Work out the finished part from the listing and answer in its coordinate system (mm). Face numbers are marked on the shaded views. A direction names the side the tool comes from. Give positions to 0.01 mm unless a question says otherwise; leave off trailing zeros. Write each loop counter-clockwise with the first axis right and the second up, starting at its lowest first coordinate (ties: lowest second). Pieces come first, ordered by that corner, then holes.
1) Given pin 1 Ø3 at (x, z) = (-38.5, -9) entering from -Y; pin 2 Ø3 at (x, z) = (14, 1) entering from +Y; pin 3 Ø0.5 at (y, z) = (13.5, -7.5) entering from -X; pin 4 Ø3 at (x, z) = (-38, 8) entering from -Y, each flat-ended and moving along its own axis, determine where each tip first touches the part or whether it passes through.
2) Determine the mould class of the marked faces 1, 2 and 3 for opening direction Z: pulls with the +Z half, pulls with the -Z half, needs draft (parallel to the pull), parting line crosses it, or undercut.
3) Find section B-B (z = 11). Determine the outline of the cut face in (x, y).
4) Find section A-A (y = 2.5). Determine the outline of the cut face in (x, z), plus the area to 3 significant figures.
5) A tool of negligible diameter and unlimited length cuts with its end or side. For the marked faces 4 and 5, from which of +Z, -Z, +X, -X, +Y, -Y can it reach the whole face along a straight path? Write none if from no direction.
6) Find section D-D (z = -8). Determine the outline of the cut face in (x, y), plus the area to 3 significant figures.
7) Straight lines are drawn through the part: probe 1 along X at (y, z) = (2.1, 8); probe 2 along Z at (x, y) = (24, 4); probe 3 along Y at (x, z) = (-5, 2). For each, find the intervals that lie inside material, in ascending order.
8) Find section C-C (x = 10). Determine the outline of the cut face in (y, z).
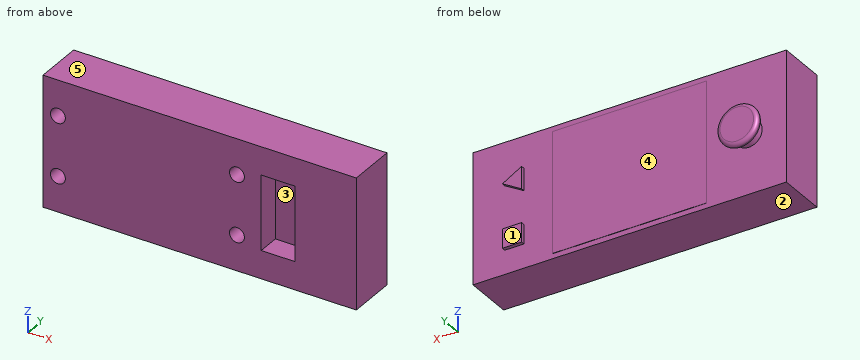
```python
from build123d import *

# Parameters (mm, degrees)
SKETCH_1_W          = 84
SKETCH_1_H          = 35
EXTRUDE_1_DEPTH     = 13
SKETCH_2_R          = 3.636879205
EXTRUDE_2_DEPTH     = 3
EXTRUDE_2_TAPER     = 10
SKETCH_2_3_W        = 5.141866658
SKETCH_2_3_H        = 5.141866659
EXTRUDE_3_DEPTH     = 1
SKETCH_2_4_W        = 41.257358664
SKETCH_2_4_H        = 32.32030471
EXTRUDE_4_DEPTH     = 0.1
SKETCH_4_R          = 5.5
EXTRUDE_5_DEPTH     = 2
FILLET_1_R          = 1
SKETCH_5_R          = 2
SKETCH_5_W          = 9
SKETCH_5_H          = 20
CUT_EXTRUDE_1_DEPTH = 6


with BuildPart() as part:
    # 草图1 → 凸台-拉伸1 (new body)
    with BuildSketch(Plane(origin=(0, 0, 0), x_dir=(1, 0, 0), z_dir=(0, 1, 0))):
        Rectangle(SKETCH_1_W, SKETCH_1_H)
    extrude(amount=EXTRUDE_1_DEPTH)

    # 草图2 → 凸台-拉伸2 (add)
    with BuildSketch(Plane(origin=(0, 13, 0), x_dir=(1, 0, 0), z_dir=(0, 1, 0))):
        with Locations((-31.891815821, 1.407892061)):
            Circle(SKETCH_2_R)
    extrude(amount=EXTRUDE_2_DEPTH, taper=EXTRUDE_2_TAPER)

    # 草图2<3> → 凸台-拉伸3 (add)
    with BuildSketch(Plane(origin=(0, 13, 0), x_dir=(1, 0, 0), z_dir=(0, 1, 0))):
        with Locations((30.912412648, 8.508565066)):
            Rectangle(SKETCH_2_3_W, SKETCH_2_3_H)
        Polygon((28.341479319, -3.030186335), (28.341479319, -8.967502534), (33.483345977, -5.998844435), align=None)
    extrude(amount=EXTRUDE_3_DEPTH)

    # 草图2<4> → 凸台-拉伸4 (add)
    with BuildSketch(Plane(origin=(0, 13, 0), x_dir=(1, 0, 0), z_dir=(0, 1, 0))):
        Rectangle(SKETCH_2_4_W, SKETCH_2_4_H)
    extrude(amount=EXTRUDE_4_DEPTH)

    # 草图4 → 凸台-拉伸5 (add)
    with BuildSketch(Plane(origin=(0, 16, 0), x_dir=(1, 0, 0), z_dir=(0, 1, 0))):
        with Locations(Location((-31.891815821, 1.407892061, 0), (0, 0, 270))):
            Circle(SKETCH_4_R)
    extrude(amount=EXTRUDE_5_DEPTH)

    # 圆角1
    fillet_1_edges = [part.edges().sort_by_distance(p)[0] for p in [
        (-31.891815821, 16, -6.907892061),
        (-31.891815821, 18, -6.907892061),
    ]]
    fillet(fillet_1_edges, radius=FILLET_1_R - 0.0001)  # a hair under: the kernel refuses the full size

    # 草图5 → 切除-拉伸1 (cut)
    with BuildSketch(Plane.XZ):
        with Locations(Location((-38, 8, 0), (0, 0, 270))):
            Circle(SKETCH_5_R)
        with Locations(Location((-38, -8, 0), (0, 0, 270))):
            Circle(SKETCH_5_R)
        with Locations(Location((10, 8, 0), (0, 0, 270))):
            Circle(SKETCH_5_R)
        with Locations(Location((10, -8, 0), (0, 0, 270))):
            Circle(SKETCH_5_R)
        with Locations((21, 0)):
            Rectangle(SKETCH_5_W, SKETCH_5_H)
    extrude(amount=-CUT_EXTRUDE_1_DEPTH, mode=Mode.SUBTRACT)


solid = part.part
```
Results:
1. pin 1: stops at y = 0
1. pin 2: stops at y = 13.1
1. pin 3: stops at x = 28.34
1. pin 4: stops at y = 6
2. face 1: needs draft
2. face 2: pulls with the -Z half
2. face 3: undercut
3. outline: (-42, 0) - (42, 0) - (42, 13) - (20.63, 13) - (20.63, 13.1) - (-20.63, 13.1) - (-20.63, 13) - (-42, 13) - close
4. outline: (-42, -17.5) - (42, -17.5) - (42, 17.5) - (-42, 17.5) - close; hole circle Ø4 at (-38, -8); hole circle Ø4 at (-38, 8); hole circle Ø4 at (10, -8); hole circle Ø4 at (10, 8); hole (16.5, -10) - (25.5, -10) - (25.5, 10) - (16.5, 10) - close
4. area: 2,710 mm2
5. face 4: +Z, -Z, +Y
5. face 5: +Z, +X, -X, +Y, -Y
6. outline: (-42, 0) - (-40, 0) - (-40, 6) - (-36, 6) - (-36, 0) - (8, 0) - (8, 6) - (12, 6) - (12, 0) - (16.5, 0) - (16.5, 6) - (25.5, 6) - (25.5, 0) - (42, 0) - (42, 13) - (33.48, 13) - (33.48, 14) - (28.34, 14) - (28.34, 13) - (20.63, 13) - (20.63, 13.1) - (-20.63, 13.1) - (-20.63, 13) - (-42, 13) - close
6. area: 999 mm2
7. probe 1: x = -42 to -40, -36 to 8, 12 to 16.5, 25.5 to 42
7. probe 2: z = -17.5 to -10, 10 to 17.5
7. probe 3: y = 0 to 13.1
8. outline: (0, -17.5) - (13, -17.5) - (13, -16.16) - (13.1, -16.16) - (13.1, 16.16) - (13, 16.16) - (13, 17.5) - (0, 17.5) - (0, 10) - (6, 10) - (6, 6) - (0, 6) - (0, -6) - (6, -6) - (6, -10) - (0, -10) - close
